```python
from build123d import *

# Parameters (mm, degrees)
BOSS_EXTRUDE1_DEPTH                  = 2.5
TAP_DRILL_FOR_M2_TAP1_D              = 1.6
TAP_DRILL_FOR_M2_TAP1_DEPTH          = 12
TAP_DRILL_FOR_M2_TAP1_CSINK_D        = 1.65
TAP_DRILL_FOR_M2_TAP1_CSINK_ANGLE    = 90
TAP_DRILL_FOR_M2_TAP1_TIP            = 0.480688495
F_6_2_6_2_DIAMETER_HOLE1_D           = 6.2
F_6_2_6_2_DIAMETER_HOLE1_CSINK_D     = 6.25
F_6_2_6_2_DIAMETER_HOLE1_CSINK_ANGLE = 90


with BuildPart() as part:
    # Sketch1 → Boss-Extrude1 (new, symmetric)
    with BuildSketch(Plane(origin=(0, 0, 0), x_dir=(1, 0, 0), z_dir=(0, 1, 0))):
        Polygon((45, 15), (35, 15), (35, 10), (25, 10), (25, 15), (15, 15), (15, 10), (5, 10), (5, 15), (-5, 15), (-5, 10), (-15, 10), (-15, 15), (-25, 15), (-25, 10), (-35, 10), (-35, 15), (-45, 15), (-45, 10), (-55, 10), (-55, 5), (-60, 5), (-60, -5), (-55, -5), (-55, -10), (-45, -10), (-45, -15), (-35, -15), (-35, -10), (-25, -10), (-25, -15), (-15, -15), (-15, -10), (-5, -10), (-5, -15), (5, -15), (5, -10), (15, -10), (15, -15), (25, -15), (25, -10), (35, -10), (35, -15), (45, -15), (45, -10), (55, -10), (55, -5), (60, -5), (60, 5), (55, 5), (55, 10), (45, 10), align=None)
    extrude(amount=BOSS_EXTRUDE1_DEPTH, both=True)

    # Tap Drill for M2 Tap1
    with Locations(Plane.XY.offset(15)):
        with Locations((-3, 0), (3, 0)):
            CounterSinkHole(TAP_DRILL_FOR_M2_TAP1_D / 2, TAP_DRILL_FOR_M2_TAP1_CSINK_D / 2, depth=TAP_DRILL_FOR_M2_TAP1_DEPTH, counter_sink_angle=TAP_DRILL_FOR_M2_TAP1_CSINK_ANGLE)
            with Locations((0, 0, -(TAP_DRILL_FOR_M2_TAP1_DEPTH + TAP_DRILL_FOR_M2_TAP1_TIP / 2))):  # 118° drill point
                Cone(0, TAP_DRILL_FOR_M2_TAP1_D / 2, TAP_DRILL_FOR_M2_TAP1_TIP, mode=Mode.SUBTRACT)

    # Ø6.2 (6.2) Diameter Hole1 (through all)
    with Locations(Plane(origin=(0, 2.5, 0), x_dir=(1, 0, 0), z_dir=(0, 1, 0))):
        with Locations((-45, -4.5), (45, -4.5)):
            CounterSinkHole(F_6_2_6_2_DIAMETER_HOLE1_D / 2, F_6_2_6_2_DIAMETER_HOLE1_CSINK_D / 2, counter_sink_angle=F_6_2_6_2_DIAMETER_HOLE1_CSINK_ANGLE)


solid = part.part
```
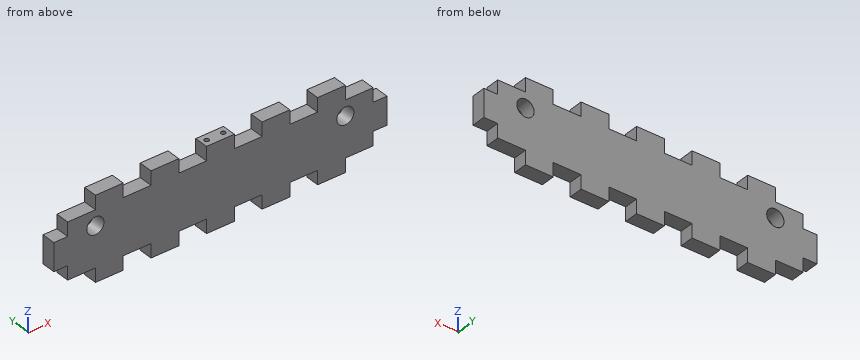
Input: part model. Units: mm. Frame: model coordinates. Give positions to 0.01 mm unless a question says otherwise; leave off trailing zeros. Loops run counter-clockwise (first coordinate to the right, second up) from the corner with the lowest first, then second, coordinate; pieces in that order, holes last. Notation, with made-up numbers: (49.5, -17.5) -> (68.5, -17.5) arc R25 ccw to (68.5, -5.5) -> close; hole circle Ø1 at (63, 58). An arc over 180 degrees is marked (long way). Use a Markdown table: item, result.
Q1. Section query B-B, the plane x = 9.5. Return the cut outline in (y, z).
Entries:
| item | result |
|---|---|
| outline | (-2.5, -10) -> (2.5, -10) -> (2.5, 10) -> (-2.5, 10) -> close |
Q2. Section query A-A, the plane y = 1.7. State how many separate pieces and enclosed holes the cut face has, plus the area to 3 significant figures.
Entries:
| item | result |
|---|---|
| separate pieces | 1 |
| enclosed holes | 2 |
| area | 2,740 mm² |
Q3. First-contact query: P1, Ø2.5, axis at y = -1, z = -11.5, coming from the -X side; P2, Ø2.5, axis at y = 0, z = -13, coming from the +X side; P3, Ø2.5, axis at y = 0.5, z = 6.5, coming from the +X side; P4, Ø5, axis at x = 45, z = 4.5, coming from the -Y side. Flat tips, straight axial feed; report the tip coordinate or a pass-through.
Entries:
| item | result |
|---|---|
| P1 | stops at x = -45 |
| P2 | stops at x = 45 |
| P3 | stops at x = 55 |
| P4 | passes through |
Q4. Ray query, probe 1 along X at (y, z) = (0, 8); probe 2 along X at (y, z) = (-1.35, -13); probe 3 along X at (y, z) = (0.25, 2). Return the intervals inside material, ascending. Write a range as from..to.
Entries:
| item | result |
|---|---|
| probe 1 | x = -55..-3.8, -2.2..2.2, 3.8..55 |
| probe 2 | x = -45..-35, -25..-15, -5..5, 15..25, 35..45 |
| probe 3 | x = -60..-46.83, -43.17..43.17, 46.83..60 |
